Verification items for the finished model (mm, model axes). Face numbers are marked on the shaded views. A direction names the side the tool comes from. Give positions to 0.01 mm unless a question says otherwise; leave off trailing zeros. Loops run counter-clockwise (first coordinate to the right, second up) from the corner with the lowest first, then second, coordinate; pieces in that order, holes last. Notation, with made-up numbers: M 83,8.25 L 87,8.25 A16 ccw 87,28.25 Z; hole C 66.5,66 d5. An arc over 180 degrees is marked long. Use CSV: the item, a comma, the result in double quotes.
from build123d import *

# Parameters (mm, degrees)
SKETCH_1_R      = 1.5
EXTRUDE_1_DEPTH = 1.6
SKETCH_2_W      = 28
SKETCH_2_H      = 12
EXTRUDE_2_DEPTH = 10
FILLET_1_R      = 3


with BuildPart() as part:
    # 草图1 → 凸台-拉伸1 (new body)
    with BuildSketch(Plane.XY):
        with BuildLine():
            Line((-30, 8), (-30, -8))
            ThreePointArc((-30, -8), (-29.121320344, -10.121320344), (-27, -11))
            Line((-27, -11), (27, -11))
            ThreePointArc((27, -11), (29.121320344, -10.121320344), (30, -8))
            Line((30, -8), (30, 8))
            ThreePointArc((30, 8), (29.121320344, 10.121320344), (27, 11))
            Line((27, 11), (-27, 11))
            ThreePointArc((-27, 11), (-29.121320344, 10.121320344), (-30, 8))
        make_face()
        with Locations((-25, 7)):
            Circle(SKETCH_1_R, mode=Mode.SUBTRACT)
        with Locations((25, 7)):
            Circle(SKETCH_1_R, mode=Mode.SUBTRACT)
        with Locations((25, -7)):
            Circle(SKETCH_1_R, mode=Mode.SUBTRACT)
        with Locations((-25, -7)):
            Circle(SKETCH_1_R, mode=Mode.SUBTRACT)
    extrude(amount=EXTRUDE_1_DEPTH)

    # 草图2 → 凸台-拉伸2 (add)
    with BuildSketch(Plane.XY.offset(1.6)):
        with Locations((4, -5)):
            Rectangle(SKETCH_2_W, SKETCH_2_H)
    extrude(amount=EXTRUDE_2_DEPTH)

    # 圆角1
    fillet_1_edges = [part.edges().sort_by_distance(p)[0] for p in [
        (-10, 1, 6.6),
        (-10, -11, 6.6),
        (18, -11, 6.6),
        (18, 1, 6.6),
    ]]
    fillet(fillet_1_edges, radius=FILLET_1_R)


solid = part.part
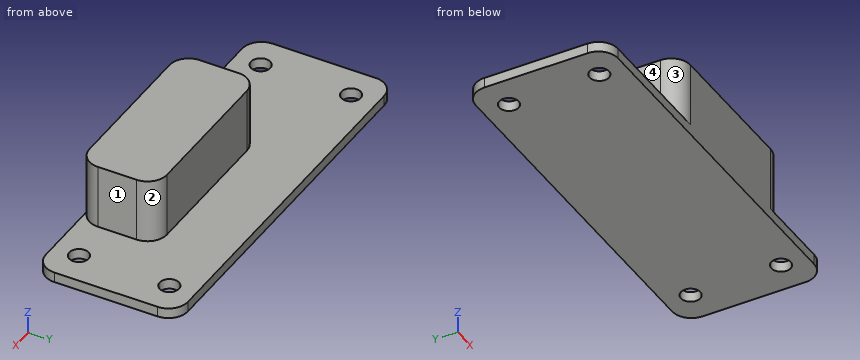
(1) Section check A-A on y = -7. Record the cut outline in (x, z), plus the area to 3 significant figures.
Calculated:
outline,"M -30,0 L -26.5,0 L -26.5,1.6 L -30,1.6 Z; M -23.5,0 L 23.5,0 L 23.5,1.6 L 18,1.6 L 18,11.6 L -10,11.6 L -10,1.6 L -23.5,1.6 Z; M 26.5,0 L 30,0 L 30,1.6 L 26.5,1.6 Z"
area,"366 mm²"
(2) Scan lines: L1, parallel to Y at x = -25, z = 0.8; L2, parallel to Y at x = -24.5, z = 1.25; L3, parallel to Z at x = -11, y = -8.25. Record each from-to range of solid material in increasing order. Write a range as from..to.
Calculated:
L1,"y = -11..-8.5, -5.5..5.5, 8.5..11"
L2,"y = -11..-8.41, -5.59..5.59, 8.41..11"
L3,"z = 0..1.6"
(3) Depth check by flat-ended pin: pin 1 Ø2 at (x, y) = (-8, 5.5) entering from +Z; pin 2 Ø5 at (y, z) = (-5, 4.5) entering from -X; pin 3 Ø1.8 at (y, z) = (-4, 5.5) entering from +X. Enter the tip coordinate at first touch or a pass-through.
Calculated:
pin 1,"stops at z = 1.6"
pin 2,"stops at x = -10"
pin 3,"stops at x = 18"
(4) Tool access check on the marked faces 1, 2, 3 and 4. Record the directions out of +Z, -Z, +X, -X, +Y, -Y that give a thin tool (end or side, any length) a straight path to the whole face; none if there is none.
Calculated:
face 1,"+Z, +X, +Y, -Y"
face 2,"+Z, +X, +Y"
face 3,"+Z, -X, -Y"
face 4,"+Z, -X, +Y, -Y"
(5) Section check D-D on y = -4.5. Record the cut outline in (x, z).
Calculated:
outline,"M -30,0 L 30,0 L 30,1.6 L 18,1.6 L 18,11.6 L -10,11.6 L -10,1.6 L -30,1.6 Z"
(6) Section check C-C on z = 2.75. Record the cut outline in (x, y).
Calculated:
outline,"M -10,-8 A3 ccw -7,-11 L 15,-11 A3 ccw 18,-8 L 18,-2 A3 ccw 15,1 L -7,1 A3 ccw -10,-2 Z"
(7) Section check B-B on x = -25. Record the cut outline in (y, z).
Calculated:
outline,"M -11,0 L -8.5,0 L -8.5,1.6 L -11,1.6 Z; M -5.5,0 L 5.5,0 L 5.5,1.6 L -5.5,1.6 Z; M 8.5,0 L 11,0 L 11,1.6 L 8.5,1.6 Z"
